Design review of the part built by this model. Coordinates are the model's own, in mm. Face numbers are marked on the shaded views. A direction names the side the tool comes from. Coordinates: 2 decimals unless noted, no trailing zeros. Loops run counter-clockwise (first coordinate to the right, second up) from the corner with the lowest first, then second, coordinate; pieces in that order, holes last. Notation, with made-up numbers: M -23,35 L -5,35 A26 ccw -5,74 Z; hole C -9,-29 d6. An arc over 180 degrees is marked long. Put each result on its own line as item: value. Start each with the question number.
(1) Take a section at B-B, the plane z = 0. Give the boundary of the cut face in (x, y), then the cut area to 3 significant figures.
(2) Take a section at A-A, the plane y = 0. Give the boundary of the cut face in (x, z), then the cut area to 3 significant figures.
(3) For probe 1 along Z at (x, y) = (8, 0); probe 2 along Z at (x, y) = (15, -0.5); probe 3 along Z at (x, y) = (10.75, -0.75), list the stretches that pass through material, from the lowest coordinate up. Write a range as [from, to].
(4) Clearance check with flat-ended pins moving along their axes: pin 1 (2 mm diameter, centred on x = 15, y = 2.5, fed in from -Z); pin 2 (4 mm diameter, centred on x = 5, z = -3, fed in from +Y); pin 3 (0.8 mm diameter, centred on y = 2, z = 0, fed in from +X). State where each tip first meets the part, or that it passes through.
(5) The part is to be moulded in two halves that separate along Z. For the marked faces 1, 2 and 3, say which applies: +Z half, -Z half, draft (parallel to the pull), parting line (faces both ways), or undercut.
(6) For the marked faces 4 and 5, list the 3-axis set-ups (+Z, -Z, +X, -X, +Y, -Y) from which the entire face can be reached by the end or side of a thin tool; tool diameter is ignored.
(7) Take a section at C-C, the plane x = 12.5. Give the boundary of the cut face in (y, z).
Solid Edge part; units mm, degrees
sketch "Sketch1" plane through (0, 0, 0) normal (0, 0, 1) x (1, 0, 0)
  line L0 (16, 0) -> (16, 6)
  line L1 (16, 6) -> (13, 3)
  line L2 (13, 3) -> (0, 3)
  line L3 (0, 3) -> (0, 0)
  line L4 (0, 0) -> (16, 0)
revolve "RevolvedProtrusion1" add sketch "Sketch1" angle 360 about axis through (0, 0, 0) along (1, 0, 0)
cosmetic_thread "Thread1"
sketch "Sketch2" plane through (16, 0, 0) normal (1, 0, 0) x (0, 1, 0)
  line L0 (6, 0.8) -> (-6, 0.8)
  line L1 (-6, 0.8) -> (-6, -0.8)
  line L2 (-6, -0.8) -> (6, -0.8)
  line L3 (6, -0.8) -> (6, 0.8)
extrude "Cutout1" cut sketch "Sketch2" against normal blind 1.9
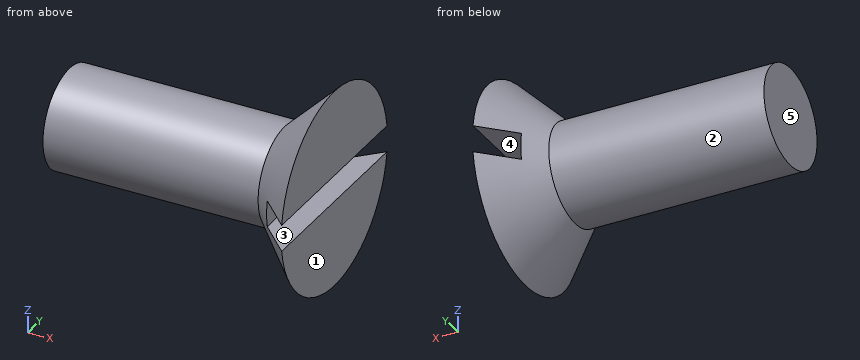
Computed values:
1. outline: M 0,-3 L 13,-3 L 14.1,-4.1 L 14.1,4.1 L 13,3 L 0,3 Z
1. area: 85.8 mm^2
2. outline: M 0,-3 L 13,-3 L 16,-6 L 16,-0.8 L 14.1,-0.8 L 14.1,0.8 L 16,0.8 L 16,6 L 13,3 L 0,3 Z
2. area: 102 mm^2
3. probe 1: z = [-3, 3]
3. probe 2: z = [-4.97, -0.8], [0.8, 4.97]
3. probe 3: z = [-2.9, 2.9]
4. pin 1: stops at z = -5.53
4. pin 2: stops at y = 2.83
4. pin 3: stops at x = 14.1
5. face 1: draft
5. face 2: parting line
5. face 3: undercut
6. face 4: +X, +Y, -Y
6. face 5: +Z, -Z, -X, +Y, -Y
7. outline: C 0,0 d6
